For this review, take the finished solid that the model builds, in its own axes (mm). Face numbers are marked on the shaded views. Round coordinates to 2 decimals unless told otherwise and drop trailing zeros. Order: outer loops, then holes, each group sorted by start corner. A loop starts at its lowest first (then second) coordinate and runs counter-clockwise, first axis right, second up.
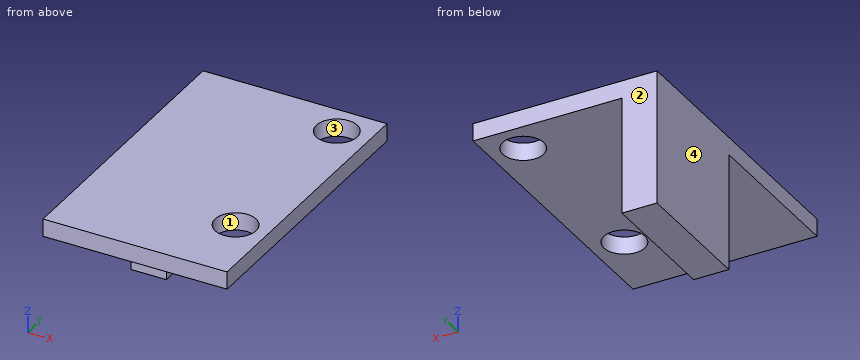
```python
from build123d import *

# Parameters (mm, degrees)
ESQUISSE1_W        = 15.7
ESQUISSE1_H        = 24.5
ESQUISSE1_R        = 1.75
BOSS_EXTRU_1_DEPTH = 1.5
ESQUISSE2_W        = 3
ESQUISSE2_H        = 11
BOSS_EXTRU_2_DEPTH = 10


with BuildPart() as part:
    # Esquisse1 → Boss.-Extru.1 (new body)
    with BuildSketch(Plane.XY):
        with Locations((-7.85, 12.25)):
            Rectangle(ESQUISSE1_W, ESQUISSE1_H)
        with Locations((-2.75, 21.75)):
            Circle(ESQUISSE1_R, mode=Mode.SUBTRACT)
        with Locations((-2.75, 6.25)):
            Circle(ESQUISSE1_R, mode=Mode.SUBTRACT)
    extrude(amount=BOSS_EXTRU_1_DEPTH)

    # Esquisse2 → Boss.-Extru.2 (add)
    with BuildSketch(Plane(origin=(0, 0, 0), x_dir=(-1, 0, 0), z_dir=(0, 0, -1))):
        with Locations((14.2, 19)):
            Rectangle(ESQUISSE2_W, ESQUISSE2_H)
    extrude(amount=BOSS_EXTRU_2_DEPTH)


solid = part.part
```
Q1. Mouldability with a two-part tool opening along Y and no side actions: class the marked faces 1, 2, 3 and 4 as +Y half, -Y half, draft (parallel to the pull), parting line (faces both ways), or undercut.
Q2. Take a section at D-D, the plane y = 21.75. State the section outline as (x, z) points, plus the area to 3 significant figures.
Q3. Take a section at B-B, the plane x = -2.75. State the section outline as (y, z) points.
Q4. Take a section at A-A, the plane y = 6.25. State the section outline as (x, z) points, plus the area to 3 significant figures.
Q5. Wall thickness on line 1 (Y direction, x = -2.75, z = 0.3); line 2 (Z direction, x = -14, y = 10.75); line 3 (X direction, y = 18, z = -4): over which ranges is each line inside the solid? List them lowest first.
Q6. Take a section at C-C, the plane z = 0.75. State the section outline as (x, y) points, plus the area to 3 significant figures.
Q7. Clearance check with flat-ended pins moving along their axes: pin 1 (3.5 mm diameter, centred on x = -15, z = -6.5, fed in from -Y); pin 2 (4.5 mm diameter, centred on x = -6.5, y = 16, fed in from -Z); pin 3 (4 mm diameter, centred on x = -2.75, y = 6.25, fed in from +Z); pin 4 (5 mm diameter, centred on y = 12, z = -6, fed in from +X). State where each tip first meets the part, or that it passes through.
Working result:
1. face 1: undercut
1. face 2: +Y half
1. face 3: undercut
1. face 4: draft
2. outline: (-15.7, -10) - (-12.7, -10) - (-12.7, 0) - (-4.5, 0) - (-4.5, 1.5) - (-15.7, 1.5) - close; (-1, 0) - (0, 0) - (0, 1.5) - (-1, 1.5) - close
2. area: 48.3 mm2
3. outline: (0, 0) - (4.5, 0) - (4.5, 1.5) - (0, 1.5) - close; (8, 0) - (20, 0) - (20, 1.5) - (8, 1.5) - close; (23.5, 0) - (24.5, 0) - (24.5, 1.5) - (23.5, 1.5) - close
4. outline: (-15.7, 0) - (-4.5, 0) - (-4.5, 1.5) - (-15.7, 1.5) - close; (-1, 0) - (0, 0) - (0, 1.5) - (-1, 1.5) - close
4. area: 18.3 mm2
5. line 1: y = 0 to 4.5, 8 to 20, 23.5 to 24.5
5. line 2: z = 0 to 1.5
5. line 3: x = -15.7 to -12.7
6. outline: (-15.7, 0) - (0, 0) - (0, 24.5) - (-15.7, 24.5) - close; hole circle Ø3.5 at (-2.75, 6.25); hole circle Ø3.5 at (-2.75, 21.75)
6. area: 365 mm2
7. pin 1: stops at y = 13.5
7. pin 2: stops at z = 0
7. pin 3: stops at z = 1.5
7. pin 4: stops at x = -12.7
